```python
from build123d import *

# Parameters (mm, degrees)
SKETCH1_W                      = 30
SKETCH1_H                      = 40.9
SKETCH1_R                      = 12
BOSS_EXTRUDE1_DEPTH            = 10
BOSS_EXTRUDE2_START            = 2
SKETCH2_R                      = 12
SKETCH2_R_2                    = 10
BOSS_EXTRUDE2_DEPTH            = 2
SKETCH3_W                      = 2.5
SKETCH3_H                      = 9.078432584
CUT_EXTRUDE1_DEPTH             = 29.365648239
CBORE_FOR_M3_SHCS1_D           = 3.2
CBORE_FOR_M3_SHCS1_DEPTH       = 13.75
CBORE_FOR_M3_SHCS1_CBORE_D     = 6.5
CBORE_FOR_M3_SHCS1_CBORE_DEPTH = 3
TAP_DRILL_FOR_M3X0_5_TAP1_D    = 2.5
CHAMFER1_SIZE                  = 0.5
SKETCH8_W                      = 30
SKETCH8_H                      = 10
BOSS_EXTRUDE3_DEPTH            = 8
M5_CLEARANCE_HOLE1_D           = 5.3


with BuildPart() as part:
    # Sketch1 → Boss-Extrude1 (new body)
    with BuildSketch(Plane.XY):
        with Locations((0, -1.45)):
            Rectangle(SKETCH1_W, SKETCH1_H)
        Circle(SKETCH1_R, mode=Mode.SUBTRACT)
    extrude(amount=BOSS_EXTRUDE1_DEPTH)

    # Sketch2 → Boss-Extrude2 (add)
    with BuildSketch(Plane(origin=(0, 0, 10), x_dir=(-1, 0, 0), z_dir=(0, 0, -1)).offset(BOSS_EXTRUDE2_START)):
        Circle(SKETCH2_R)
        Circle(SKETCH2_R_2, mode=Mode.SUBTRACT)
    extrude(amount=-BOSS_EXTRUDE2_DEPTH)

    # Sketch3 → Cut-Extrude1 (cut, through all)
    with BuildSketch(Plane.XY.offset(10)):
        with Locations((0, 14.460783708)):
            Rectangle(SKETCH3_W, SKETCH3_H)
    extrude(amount=-CUT_EXTRUDE1_DEPTH, mode=Mode.SUBTRACT)

    # CBORE for M3 SHCS1
    with Locations(Plane(origin=(15, 0, 0), x_dir=(0, 0, -1), z_dir=(1, 0, 0))):
        with Locations((-5, 14)):
            CounterBoreHole(CBORE_FOR_M3_SHCS1_D / 2, CBORE_FOR_M3_SHCS1_CBORE_D / 2, CBORE_FOR_M3_SHCS1_CBORE_DEPTH, depth=CBORE_FOR_M3_SHCS1_DEPTH)

    # Tap Drill for M3x0.5 Tap1 (through all)
    with Locations(Plane.ZY.offset(15)):
        with Locations((5, 14)):
            Hole(TAP_DRILL_FOR_M3X0_5_TAP1_D / 2)

    # Chamfer1
    chamfer1_edges = [part.edges().sort_by_distance(p)[0] for p in [
        (0, -10, 10),
        (0, -12, 0),
    ]]
    chamfer(chamfer1_edges, length=CHAMFER1_SIZE)

    # Sketch8 → Boss-Extrude3 (add)
    with BuildSketch(Plane.XZ.offset(21.9)):
        with Locations((0, 15)):
            Rectangle(SKETCH8_W, SKETCH8_H)
    extrude(amount=-BOSS_EXTRUDE3_DEPTH)

    # M5 Clearance Hole1 (through all)
    with Locations(Plane(origin=(0, -13.9, 0), x_dir=(1, 0, 0), z_dir=(0, 1, 0))):
        with Locations((-10, -15), (10, -15)):
            Hole(M5_CLEARANCE_HOLE1_D / 2)


with BuildPart() as body_2:
    # Mirror1: mirrored copy
    add(part.part.mirror(Plane(origin=(0, 0, 0), x_dir=(0, 0, 1), z_dir=(1, 0, 0))))


solid = body_2.part
```
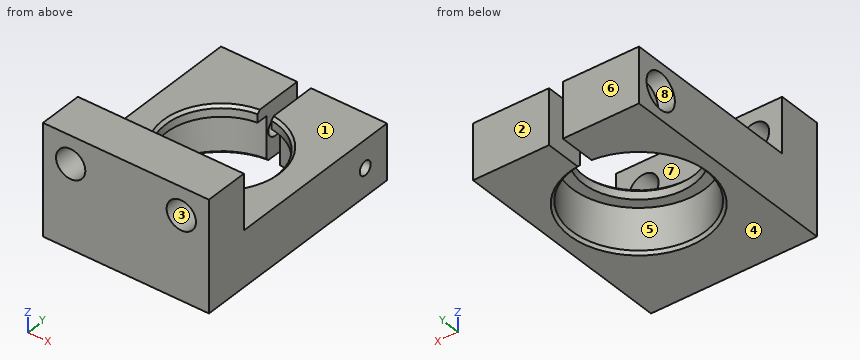
Geometry check sheet. Reference: the model listing, model coordinates, mm. Face numbers are marked on the shaded views. A direction names the side the tool comes from. Coordinates: 2 decimals unless noted, no trailing zeros. Order: outer loops, then holes, each group sorted by start corner. A loop starts at its lowest first (then second) coordinate and runs counter-clockwise, first axis right, second up.
Item 1: Section check A-A (z = 15). Enter the section's corners in (x, y), plus the area to 3 significant figures.
Item 2: Section check C-C (y = 14). Enter the section's corners in (x, z), plus the area to 3 significant figures.
Item 3: Mould release check, pull along Z, two halves, no side actions. Record for the marked faces 1, 2, 3 and 4: released by +Z, released by -Z, zero draft, split by the parting line, or undercut.
Item 4: Tool access check on the marked faces 5, 6, 7 and 8. Record the directions out of +Z, -Z, +X, -X, +Y, -Y that give a thin tool (end or side, any length) a straight path to the whole face; none if there is none.
Item 5: Section check B-B (y = 0). Enter the section's corners in (x, z), plus the area to 3 significant figures.
Item 6: Depth check by flat-ended pin: pin 1 (5 mm diameter, centred on x = 5.5, z = 16.5, fed in from +Y); pin 2 (8 mm diameter, centred on x = 7, y = 1, fed in from +Z); pin 3 (1 mm diameter, centred on x = 10.5, y = -5.5, fed in from -Z). Enter the tip coordinate at first touch or a pass-through.
Item 7: Scan lines: line 1 along X through (y, z) = (-18.75, 15); line 2 along Y through (x, z) = (12.25, 5); line 3 along Y through (x, z) = (-6.25, 5.75). Record each from-to range of solid material in increasing order.
Check sheet entries:
1. outline: (-15, -21.9) - (-12.65, -21.9) - (-12.65, -13.9) - (-15, -13.9) - close; (-7.35, -21.9) - (7.35, -21.9) - (7.35, -13.9) - (-7.35, -13.9) - close; (12.65, -21.9) - (15, -21.9) - (15, -13.9) - (12.65, -13.9) - close
1. area: 155 mm2
2. outline: (-15, 0) - (-1.25, 0) - (-1.25, 3.4) - (-12, 3.4) - (-12, 1.75) - (-15, 1.75) - close; (-15, 8.25) - (-12, 8.25) - (-12, 6.6) - (-1.25, 6.6) - (-1.25, 10) - (-15, 10) - close; (1.25, 0) - (15, 0) - (15, 3.75) - (1.25, 3.75) - close; (1.25, 6.25) - (15, 6.25) - (15, 10) - (1.25, 10) - close
2. area: 187 mm2
3. face 1: released by +Z
3. face 2: zero draft
3. face 3: undercut
3. face 4: released by -Z
4. face 5: -Z
4. face 6: +Z, -Z, +X, -X, +Y
4. face 7: +Z, +X, -X, +Y
4. face 8: -X
5. outline: (-15, 0) - (-12.5, 0) - (-12, 0.5) - (-12, 8) - (-10, 8) - (-10, 9.5) - (-10.5, 10) - (-15, 10) - close; (10, 8) - (12, 8) - (12, 0.5) - (12.5, 0) - (15, 0) - (15, 10) - (10.5, 10) - (10, 9.5) - close
5. area: 67.5 mm2
6. pin 1: stops at y = -13.9
6. pin 2: stops at z = 10
6. pin 3: stops at z = 0.15
7. line 1: x = -15 to -12.65, -7.35 to 7.35, 12.65 to 15
7. line 2: y = -21.9 to 12.75, 15.25 to 19
7. line 3: y = -21.9 to -10.24, 10.24 to 12.59, 15.41 to 19
